from build123d import *

# Parameters (mm, degrees)
SKETCH1_W                      = 152.4
SKETCH1_H                      = 114.3
SKETCH1_R                      = 6.34365
BOSS_EXTRUDE1_DEPTH            = 12
TAP_DRILL_FOR_10_32_TAP1_D     = 4.0386
TAP_DRILL_FOR_10_32_TAP1_DEPTH = 12.7
TAP_DRILL_FOR_10_32_TAP1_TIP   = 1.213317848
F_1_4_CLEARANCE_HOLE1_D        = 6.5278
F_1_4_CLEARANCE_HOLE1_DEPTH    = 12.7
F_1_4_CLEARANCE_HOLE1_TIP      = 1.961148974


with BuildPart() as part:
    # Sketch1 → Boss-Extrude1 (new body)
    with BuildSketch(Plane(origin=(0, 0, 0), x_dir=(0, 0, -1), z_dir=(1, 0, 0))):
        Rectangle(SKETCH1_W, SKETCH1_H)
        with Locations((-31.75, 10.16)):
            Circle(SKETCH1_R, mode=Mode.SUBTRACT)
        with Locations((12.7, 10.16)):
            Circle(SKETCH1_R, mode=Mode.SUBTRACT)
    extrude(amount=BOSS_EXTRUDE1_DEPTH)

    # Tap Drill for #10-32 Tap1
    with Locations(Plane(origin=(0, -57.15, 0), x_dir=(-1, 0, 0), z_dir=(0, -1, 0))):
        with Locations((-6, -66.675), (-6, 0), (-6, 66.675)):
            Hole(TAP_DRILL_FOR_10_32_TAP1_D / 2, depth=TAP_DRILL_FOR_10_32_TAP1_DEPTH)
            with Locations((0, 0, -(TAP_DRILL_FOR_10_32_TAP1_DEPTH + TAP_DRILL_FOR_10_32_TAP1_TIP / 2))):  # 118° drill point
                Cone(0, TAP_DRILL_FOR_10_32_TAP1_D / 2, TAP_DRILL_FOR_10_32_TAP1_TIP, mode=Mode.SUBTRACT)

    # 1/4 Clearance Hole1
    with Locations(Plane.ZY):
        with Locations((-66.04, 46.99), (66.04, 46.99)):
            Hole(F_1_4_CLEARANCE_HOLE1_D / 2, depth=F_1_4_CLEARANCE_HOLE1_DEPTH)
            with Locations((0, 0, -(F_1_4_CLEARANCE_HOLE1_DEPTH + F_1_4_CLEARANCE_HOLE1_TIP / 2))):  # 118° drill point
                Cone(0, F_1_4_CLEARANCE_HOLE1_D / 2, F_1_4_CLEARANCE_HOLE1_TIP, mode=Mode.SUBTRACT)


solid = part.part
Input: part model. Units: mm. Frame: model coordinates. A direction names the side the tool comes from. Give positions to 0.01 mm unless a question says otherwise; leave off trailing zeros. Loops run counter-clockwise (first coordinate to the right, second up) from the corner with the lowest first, then second, coordinate; pieces in that order, holes last. Notation, with made-up numbers: (76.5, 22.25) -> (113.5, 22.25) arc R22 cw to (113.5, 37.25) -> close; hole circle Ø11 at (13, 59.25). An arc over 180 degrees is marked (long way). Answer as a JSON object with one key per item and string values. Group by question number.
Item 1: Cut plane C-C, the plane y = 46.99. Return the cut outline in (x, z), and give its area (3 significant figures).
Item 2: Cut plane B-B, the plane y = 10.16. Return the cut outline in (x, z), and give its area (3 significant figures).
Item 3: Reachability of faces 1 (the cylindrical face through (5.737, -50.711, 64.673)), 2 (the cylindrical face through (5.916, 6.3, -7.666)) from +Z, -Z, +X, -X, +Y, -Y: full face, straight path, thin tool, end or side. Return the list, or none.
Item 4: Line query: probe 1 along Z at (x, y) = (6, -47.75); probe 2 along Y at (x, z) = (7.25, -12.7); probe 3 along Y at (x, z) = (7.5, -66.04). Output: solid intervals per line, ascending.
Item 5: Pull-direction query (Y, two-part tool) for faces 3 (the flat face through (6, 57.15, 1)), 4 (the flat face through (3, -57.15, 1)), 5 (the cylindrical face through (6.084, 45.004, -63.45)); classes: released by +Y, released by -Y, zero draft, split by the parting line, or undercut.
Item 6: Cut plane A-A, the plane z = -12.7. Return the cut outline in (x, y).
Checks:
{
 "1": {"outline": "(0, -76.2) -> (12, -76.2) -> (12, -69.3) -> (0, -69.3) -> close; (0, -62.78) -> (12, -62.78) -> (12, 62.78) -> (0, 62.78) -> close; (0, 69.3) -> (12, 69.3) -> (12, 76.2) -> (0, 76.2) -> close", "area": "1,670 mm²"},
 "2": {"outline": "(0, -76.2) -> (12, -76.2) -> (12, -19.04) -> (0, -19.04) -> close; (0, -6.36) -> (12, -6.36) -> (12, 25.41) -> (0, 25.41) -> close; (0, 38.09) -> (12, 38.09) -> (12, 76.2) -> (0, 76.2) -> close", "area": "1,520 mm²"},
 "3": {"face 1": "-Y", "face 2": "+X, -X"},
 "4": {"probe 1": "z = -76.2 to -68.69, -64.66 to -2.02, 2.02 to 64.66, 68.69 to 76.2", "probe 2": "y = -57.15 to 3.82, 16.5 to 57.15", "probe 3": "y = -44.22 to 43.73, 50.25 to 57.15"},
 "5": {"face 3": "released by +Y", "face 4": "released by -Y", "face 5": "undercut"},
 "6": {"outline": "(0, -57.15) -> (12, -57.15) -> (12, 3.82) -> (0, 3.82) -> close; (0, 16.5) -> (12, 16.5) -> (12, 57.15) -> (0, 57.15) -> close"}
}
